Can you work these out from the model? Positions are in its coordinate system, mm. Round coordinates to 2 decimals unless told otherwise and drop trailing zeros. Loops run counter-clockwise (first coordinate to the right, second up) from the corner with the lowest first, then second, coordinate; pieces in that order, holes last. Notation, with made-up numbers: (69.25, -40) -> (104.25, -40) arc R12 cw to (104.25, -30) -> close; hole circle Ø3 at (-12.75, 72.5). An arc over 180 degrees is marked (long way). Answer as a JSON object with one key per item and string values.
```python
from build123d import *

# Parameters (mm, degrees)
SKETCH1_W           = 30
SKETCH1_H           = 15
SKETCH1_R           = 2.6
BOSS_EXTRUDE1_DEPTH = 23
SKETCH2_W           = 15
SKETCH2_H           = 30
BOSS_EXTRUDE2_DEPTH = 23
SKETCH3_R           = 2.25
CUT_EXTRUDE1_DEPTH  = 47.478489648
BOSS_EXTRUDE3_DEPTH = 23


with BuildPart() as part:
    # Sketch1 → Boss-Extrude1 (new body)
    with BuildSketch(Plane(origin=(0, 0, 0), x_dir=(1, 0, 0), z_dir=(0, 1, 0))):
        Rectangle(SKETCH1_W, SKETCH1_H)
        with Locations(Location((0, 0, 0), (0, 0, 270))):
            Circle(SKETCH1_R, mode=Mode.SUBTRACT)
        with Locations(Location((10, 0, 0), (0, 0, 270))):
            Circle(SKETCH1_R, mode=Mode.SUBTRACT)
        with Locations(Location((-10, 0, 0), (0, 0, 270))):
            Circle(SKETCH1_R, mode=Mode.SUBTRACT)
    extrude(amount=BOSS_EXTRUDE1_DEPTH)

    # Sketch2 → Boss-Extrude2 (add)
    with BuildSketch(Plane(origin=(0, 23, 0), x_dir=(1, 0, 0), z_dir=(0, 1, 0))):
        with Locations((0, 22.5)):
            Rectangle(SKETCH2_W, SKETCH2_H)
    extrude(amount=-BOSS_EXTRUDE2_DEPTH)

    # Sketch3 → Cut-Extrude1 (cut, through all)
    with BuildSketch(Plane(origin=(0, 23, 0), x_dir=(1, 0, 0), z_dir=(0, 1, 0))):
        with Locations(Location((0, 32.5, 0), (0, 0, 270))):
            Circle(SKETCH3_R)
        with Locations(Location((0, 22.5, 0), (0, 0, 270))):
            Circle(SKETCH3_R)
        with Locations(Location((0, 12.5, 0), (0, 0, 270))):
            Circle(SKETCH3_R)
    extrude(amount=-CUT_EXTRUDE1_DEPTH, mode=Mode.SUBTRACT)

    # Sketch4 → Boss-Extrude3 (add)
    with BuildSketch(Plane(origin=(0, 23, 0), x_dir=(1, 0, 0), z_dir=(0, 1, 0))):
        Polygon((-7.5, 37.5), (-15, 7.5), (-7.5, 7.5), align=None)
        Polygon((7.5, 37.5), (7.5, 7.5), (15, 7.5), align=None)
    extrude(amount=-BOSS_EXTRUDE3_DEPTH)


solid = part.part
```
Q1. I want a section at B-B, the plane z = -22.5. Write out the boundary of the cut face in (x, y), then the cut area to 3 significant figures.
Determined:
{"outline": "(-11.25, 0) -> (-2.25, 0) -> (-2.25, 23) -> (-11.25, 23) -> close; (2.25, 0) -> (11.25, 0) -> (11.25, 23) -> (2.25, 23) -> close", "area": "414 mm²"}
Q2. I want a section at D-D, the plane z = 0. Write out the boundary of the cut face in (x, y).
Determined:
{"outline": "(-15, 0) -> (-12.6, 0) -> (-12.6, 23) -> (-15, 23) -> close; (-7.4, 0) -> (-2.6, 0) -> (-2.6, 23) -> (-7.4, 23) -> close; (2.6, 0) -> (7.4, 0) -> (7.4, 23) -> (2.6, 23) -> close; (12.6, 0) -> (15, 0) -> (15, 23) -> (12.6, 23) -> close"}
Q3. I want a section at C-C, the plane y = 14. Write out the boundary of the cut face in (x, z), then the cut area to 3 significant figures.
Determined:
{"outline": "(-15, -7.5) -> (-7.5, -37.5) -> (7.5, -37.5) -> (15, -7.5) -> (15, 7.5) -> (-15, 7.5) -> close; hole circle Ø5.2 at (-10, 0); hole circle Ø5.2 at (0, 0); hole circle Ø4.5 at (0, -32.5); hole circle Ø4.5 at (0, -22.5); hole circle Ø4.5 at (0, -12.5); hole circle Ø5.2 at (10, 0)", "area": "1,010 mm²"}
Q4. I want a section at A-A, the plane x = 0. Write out the boundary of the cut face in (y, z).
Determined:
{"outline": "(0, -37.5) -> (23, -37.5) -> (23, -34.75) -> (0, -34.75) -> close; (0, -30.25) -> (23, -30.25) -> (23, -24.75) -> (0, -24.75) -> close; (0, -20.25) -> (23, -20.25) -> (23, -14.75) -> (0, -14.75) -> close; (0, -10.25) -> (23, -10.25) -> (23, -2.6) -> (0, -2.6) -> close; (0, 2.6) -> (23, 2.6) -> (23, 7.5) -> (0, 7.5) -> close"}
Q5. I'm going to push flat-ended pins straight in: pin 1 (4 mm diameter, centred on y = 7, z = -19, fed in from -X) (3 decimals); pin 2 (2.5 mm diameter, centred on x = 0, z = -32.5, fed in from +Y); pin 3 (10 mm diameter, centred on y = 13, z = -19, fed in from -X) (3 decimals); pin 4 (6 mm diameter, centred on y = 17.5, z = -17.5, fed in from +X). Where does each tip first touch, or does it pass through?
Determined:
{"pin 1": "x = -12.625", "pin 2": "through", "pin 3": "x = -13.375", "pin 4": "x = 13.25"}
Q6. If I drill on L1, parallel to X at y = 11.25, z = 0; L2, parallel to Z at x = 1, y = 12.5; L3, parallel to Z at x = -2, y = 4.25, over which ranges is the centre line in solid material (lowest first)? Write a range as [from, to].
Determined:
{"L1": "[-15, -12.6], [-7.4, -2.6], [2.6, 7.4], [12.6, 15]", "L2": "[-37.5, -34.52], [-30.48, -24.52], [-20.48, -14.52], [-10.48, -2.4], [2.4, 7.5]", "L3": "[-37.5, -33.53], [-31.47, -23.53], [-21.47, -13.53], [-11.47, -1.66], [1.66, 7.5]"}
Q7. We'd pull the mould along X, two halves only. Please class faces 1 (the flat face through (15, 11, 0)), 2 (the cylindrical face through (0.78, 11.34, 2.48)), 3 (the flat face through (0, 0, -15)), 4 (the cylindrical face through (-12.54, 11.34, -0.56)): pulls with the +X half, pulls with the -X half, needs draft (parallel to the pull), parting line crosses it, or undercut.
Determined:
{"face 1": "pulls with the +X half", "face 2": "undercut", "face 3": "needs draft", "face 4": "undercut"}
